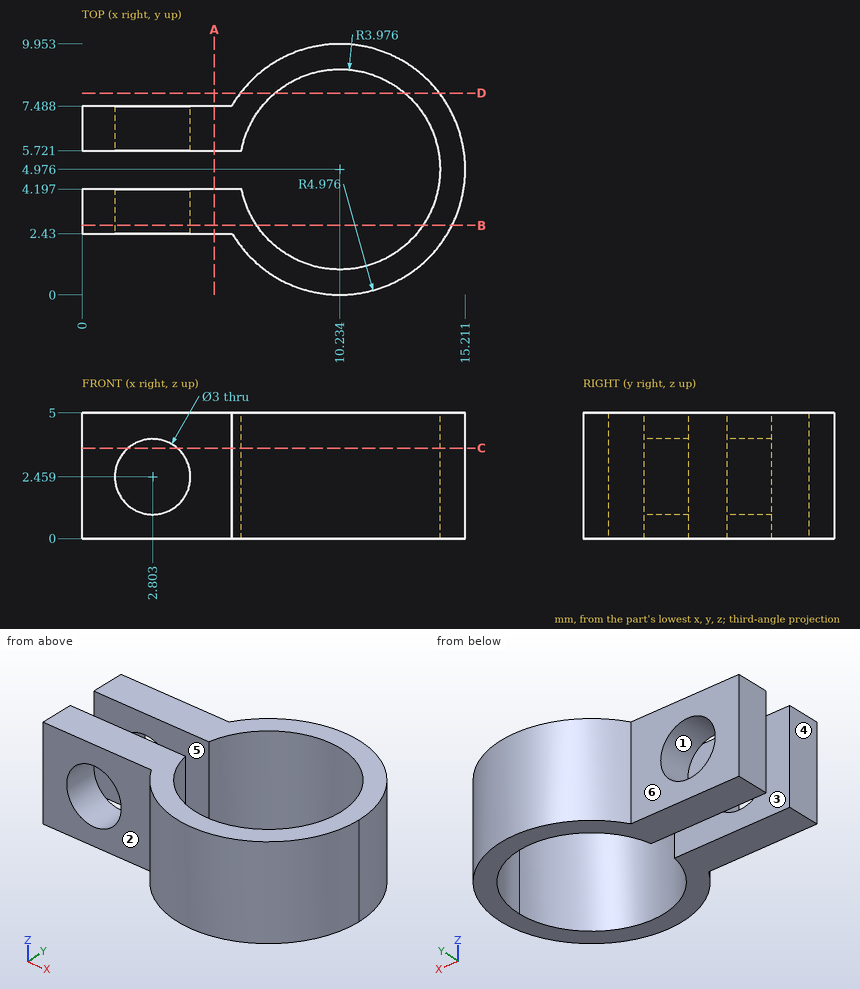
Can you work these out from the drawing? Everything is in mm from the part's minimum corner. A direction names the side the tool comes from. Coordinates: 2 decimals unless noted, no trailing zeros. Loops run counter-clockwise (first coordinate to the right, second up) from the corner with the lowest first, then second, coordinate; pieces in that order, holes last. Notation, with made-up numbers: M 2.5,45 L 34.5,45 A29 ccw 34.5,68 Z; hole C 73,40 d7. An arc over 180 degrees is marked long. One line per item, written item: value.
1. Please list where these lines run through material, in increasing order: probe 1 along Y at (x, z) = (2.75, 0.9); probe 2 along X at (y, z) = (3.5, 3.8) (1 decimal); probe 3 along X at (y, z) = (6.5, 3.5) (1 decimal).
Geometry says:
probe 1: y = 2.43 to 4.2, 5.72 to 7.49
probe 2: x = 0 to 2.1, 3.5 to 6.5, 13.9 to 15
probe 3: x = 0 to 1.7, 3.9 to 6.6, 13.9 to 15
2. Imagine slicing it at D-D (y = 8). List the corners of the cut face in (x, z) for me.
Geometry says:
outline: M 6.28,0 L 7.65,0 L 7.65,5 L 6.28,5 Z; M 12.82,0 L 14.19,0 L 14.19,5 L 12.82,5 Z
3. Imagine slicing it at B-B (y = 2.75). List the corners of the cut face in (x, z) for me (1 decimal).
Geometry says:
outline: M 0,0 L 6.9,0 L 6.9,5 L 0,5 Z; M 13.5,0 L 14.7,0 L 14.7,5 L 13.5,5 Z; hole C 2.8,2.5 d3
4. On a 3-axis mill with a long thin cutter (end or side, diameter ignored), from which of +Z, -Z, +X, -X, +Y, -Y can I reach the whole of each face in a straight line? I mean the marked faces 1, 2 and 3. Say none if no direction works.
Geometry says:
face 1: +Y, -Y
face 2: +Z, -Z, -X, -Y
face 3: +Z, -Z, -X
5. Imagine slicing it at C-C (z = 3.6). List the corners of the cut face in (x, y) for me (1 decimal).
Geometry says:
outline: M 0,2.4 L 1.8,2.4 L 1.8,4.2 L 0,4.2 Z; M 0,5.7 L 1.8,5.7 L 1.8,7.5 L 0,7.5 Z; M 3.8,2.4 L 6,2.4 A5 ccw long 5.9,7.5 L 3.8,7.5 L 3.8,5.7 L 6.3,5.7 A4 cw long 6.3,4.2 L 3.8,4.2 Z
6. Will these pins go through, and if not, where does the flat tip stop? pin 1 Ø4 at (x, y) = (4.5, 8.5) entering from -Z; pin 2 Ø1.5 at (y, z) = (8.5, 1.5) entering from +X (1 decimal); pin 3 Ø1.5 at (x, z) = (4.5, 3) entering from +Y; pin 4 Ø2.5 at (x, z) = (4.5, 2) entering from -Y.
Geometry says:
pin 1: stops at z = 0
pin 2: stops at x = 14.4
pin 3: stops at y = 7.49
pin 4: stops at y = 2.43
7. Imagine slicing it at A-A (x = 5.25). List the corners of the cut face in (y, z) for me.
Geometry says:
outline: M 2.43,0 L 4.2,0 L 4.2,5 L 2.43,5 Z; M 5.72,0 L 7.49,0 L 7.49,5 L 5.72,5 Z
8. Thinking about a two-plate mould opening in Y: for the marked faces 4, 5 and 6, which applies, +Y half, -Y half, draft (parallel to the pull), parting line (faces both ways), or undercut?
Geometry says:
face 4: draft
face 5: undercut
face 6: +Y half
